```python
from build123d import *

# Parameters (mm, degrees)
ESQUISSE1_W                  = 40
ESQUISSE1_H                  = 20
BOSS_EXTRU_1_DEPTH           = 4
ESQUISSE2_R                  = 2.95
BOSS_EXTRU_2_DEPTH           = 6
ENL_V_MAT_EXTRU_1_DEPTH      = 46.122056691
ENL_V_MAT_EXTRU_1_DEPTH_BACK = 46.122056691
ESQUISSE3_R                  = 2.55
ESQUISSE4_W                  = 21
ESQUISSE4_H                  = 5
BOSS_EXTRU_4_DEPTH           = 4
ESQUISSE5_W                  = 21
ESQUISSE5_H                  = 10.5
BOSS_EXTRU_5_DEPTH           = 6
ENL_V_START                  = -6
ESQUISSE6_R                  = 8.25
ESQUISSE6_R_2                = 2.95
ENL_V_MAT_EXTRU_2_DEPTH      = 6
CHANFREIN1_SIZE              = 5
ESQUISSE7_R                  = 1.65
ENL_V_MAT_EXTRU_3_DEPTH      = 16.5
CONG_1_R                     = 3
CONG_2_R                     = 1


with BuildPart() as part:
    # Esquisse1 → Boss.-Extru.1 (new body)
    with BuildSketch(Plane.XY):
        with Locations((20, 10)):
            Rectangle(ESQUISSE1_W, ESQUISSE1_H)
    extrude(amount=BOSS_EXTRU_1_DEPTH)

    # Esquisse2 → Boss.-Extru.2 (add)
    with BuildSketch(Plane.XY.offset(4)):
        with Locations(Location((6, 10, 0), (0, 0, 180))):
            Circle(ESQUISSE2_R)
    extrude(amount=BOSS_EXTRU_2_DEPTH)

    # Esquisse3 → Enlèv. mat.-Extru.1 (cut, two sides: drawn at the far end of the back side and taken through both)
    with BuildSketch(Plane.XY.offset(4).offset(-ENL_V_MAT_EXTRU_1_DEPTH_BACK)):
        with Locations((35.5, 10)):
            Circle(ESQUISSE3_R)
    extrude(amount=ENL_V_MAT_EXTRU_1_DEPTH + ENL_V_MAT_EXTRU_1_DEPTH_BACK, mode=Mode.SUBTRACT)

    # Esquisse4 → Boss.-Extru.4 (add)
    with BuildSketch(Plane.XY.offset(4)):
        with Locations((10.5, 22.5)):
            Rectangle(ESQUISSE4_W, ESQUISSE4_H)
    extrude(amount=-BOSS_EXTRU_4_DEPTH)

    # Esquisse5 → Boss.-Extru.5 (add)
    with BuildSketch(Plane.XY.offset(4)):
        with Locations((10.5, 19.75)):
            Rectangle(ESQUISSE5_W, ESQUISSE5_H)
    extrude(amount=BOSS_EXTRU_5_DEPTH)

    # Esquisse6 → Enlèv. mat.-Extru.2 (cut)
    with BuildSketch(Plane.XY.offset(10).offset(ENL_V_START)):
        with Locations((6, 10)):
            Circle(ESQUISSE6_R)
        with Locations(Location((6, 10, 0), (0, 0, 180))):
            Circle(ESQUISSE6_R_2, mode=Mode.SUBTRACT)
    extrude(amount=ENL_V_MAT_EXTRU_2_DEPTH, mode=Mode.SUBTRACT)

    # Chanfrein1
    chanfrein1_edges = [part.edges().sort_by_distance(p)[0] for p in [
        (21, 25, 5),
    ]]
    chamfer(chanfrein1_edges, length=CHANFREIN1_SIZE)

    # Esquisse7 → Enlèv. mat.-Extru.3 (cut)
    with BuildSketch(Plane(origin=(20.5, 20.5, 0), x_dir=(0, 0, -1), z_dir=(0.7071067811865471, 0.707106781186548, 0))):
        with Locations(Location((-7, 2.828427125, 0), (0, 0, 90))):
            Circle(ESQUISSE7_R)
    extrude(amount=-ENL_V_MAT_EXTRU_3_DEPTH, mode=Mode.SUBTRACT)

    # Congé1
    cong_1_edges = [part.edges().sort_by_distance(p)[0] for p in [
        (0, 25, 5),
        (21, 14.5, 7),
        (40, 20, 2),
        (40, 0, 2),
        (0, 0, 2),
    ]]
    fillet(cong_1_edges, radius=CONG_1_R)

    # Congé2
    cong_2_edges = [part.edges().sort_by_distance(p)[0] for p in [
        (0, 15.662375826, 7),
    ]]
    fillet(cong_2_edges, radius=CONG_2_R)


solid = part.part
```
Input: part model. Units: mm. Frame: model coordinates. A direction names the side the tool comes from. Coordinates: 2 decimals unless noted, no trailing zeros. Write each loop counter-clockwise with the first axis right and the second up, starting at its lowest first coordinate (ties: lowest second). Pieces come first, ordered by that corner, then holes. Notation, with made-up numbers: (-40, 56.5) -> (-25, 56.5) arc R30 ccw to (-25, 78.5) -> close; hole circle Ø9 at (62, 22). An arc over 180 degrees is marked (long way). Answer as a JSON object with one key per item and string values.
1. Material intervals for line 1 (X direction, y = 10, z = 2.7); line 2 (Y direction, x = 35.5, z = 2.1); line 3 (Y direction, x = 7, z = 9), sorted ascending. Write a range as from..to.
Result set:
{"line 1": "x = 0..32.95, 38.05..40", "line 2": "y = 0..7.45, 12.55..20", "line 3": "y = 7.22..12.78, 18.19..25"}
2. First-contact query: P1, Ø6, axis at x = 10, y = 12, coming from the +Z side; P2, Ø0.8, axis at y = 18, z = 8, coming from the +X side; P3, Ø4, axis at x = 35.5, y = 10, coming from the -Z side; P4, Ø2, axis at x = 22, y = 17, coming from the +Z side. Flat tips, straight axial feed; report the tip coordinate or a pass-through.
Result set:
{"P1": "stops at z = 10", "P2": "stops at x = 21", "P3": "passes through", "P4": "stops at z = 4"}
3. Section A-A on x = 35.5. Return the cut outline in (y, z), then the cut area to 3 significant figures.
Result set:
{"outline": "(0, 0) -> (7.45, 0) -> (7.45, 4) -> (0, 4) -> close; (12.55, 0) -> (20, 0) -> (20, 4) -> (12.55, 4) -> close", "area": "59.6 mm2"}
4. Section B-B on z = 3. Return the cut outline in (x, y), then the cut area to 3 significant figures.
Result set:
{"outline": "(0, 3) arc R3 ccw to (3, 0) -> (37, 0) arc R3 ccw to (40, 3) -> (40, 17) arc R3 ccw to (37, 20) -> (21, 20) -> (16, 25) -> (3, 25) arc R3 ccw to (0, 22) -> close; hole circle Ø5.1 at (35.5, 10)", "area": "864 mm2"}
5. Section C-C on z = 6. Return the cut outline in (x, y), then the cut area to 3 significant figures.
Result set:
{"outline": "(0, 17.78) arc R1 ccw to (1.54, 16.94) arc R8.25 cw to (10.83, 16.69) -> (17.57, 23.43) -> (16, 25) -> (3, 25) arc R3 ccw to (0, 22) -> close; (5.9, 11.76) -> (6.94, 12.8) arc R2.95 ccw (long way) to (8.8, 10.94) -> (7.76, 9.9) -> close; (12.69, 14.83) arc R8.25 cw to (12.91, 14.5) -> (18, 14.5) arc R3 ccw to (21, 17.5) -> (21, 20) -> (19.43, 21.57) -> close", "area": "165 mm2"}
6. Access query for faces 4 (the face through (0.51, 16.91, 6.96)), 5 (the face through (7.819, 18.047, 6.958)), 6 (the face through (15, 14.5, 7)), 7 (the face through (20.14, 15.4, 7.04)). Directions: +Z, -Z, +X, -X, +Y, -Y. A direction counts if a zero-diameter tool reaches every point of the face in a straight line with its end or side. Return the directions, or none.
Result set:
{"face 4": "+Z, -Y", "face 5": "+Z", "face 6": "+Z, +X, -X, -Y", "face 7": "+Z, +X, -Y"}
7. Section D-D on x = 26.5. Return the cut outline in (y, z), then the cut area to 3 significant figures.
Result set:
{"outline": "(0, 0) -> (20, 0) -> (20, 4) -> (0, 4) -> close", "area": "80.0 mm2"}
8. Mould query, pull axis Z, two halves, no side actions, for faces 1 (the face through (20, 10, 4)), 2 (the face through (6.849, 10.816, 7.023)), 3 (the face through (0, 14, 3)). Classes: released by +Z, released by -Z, zero draft, split by the parting line, or undercut.
Result set:
{"face 1": "released by +Z", "face 2": "undercut", "face 3": "zero draft"}
